Source: CAD feature listing. Evaluate the final solid. Frame: model axes, mm. A direction names the side the tool comes from. Round coordinates to 2 decimals unless told otherwise and drop trailing zeros. Write each loop counter-clockwise with the first axis right and the second up, starting at its lowest first coordinate (ties: lowest second). Pieces come first, ordered by that corner, then holes. Notation, with made-up numbers: (36.25, -16.5) - (78.25, -16.5) arc R21 ccw to (78.25, -3.5) - close; hole circle Ø7 at (17, -1). An arc over 180 degrees is marked (long way). Write item = value, one per line. Start each with the question number.
Solid Edge part; units mm, degrees
sketch "Sketch1" plane through (0, 0, 0) normal (0, 1, 0) x (-1, 0, 0)
  line L0 (-47.7348, -12.5) -> (4.2652, -12.5)
  line L1 (4.2652, -12.5) -> (4.2652, 12.5)
  line L2 (-47.7348, 12.5) -> (4.2652, 12.5)
  line L3 (-47.7348, 12.5) -> (-47.7348, -12.5)
  dimension "D1" = 4.2652
  dimension "D2" = 47.7348
extrude "Protrusion1" add sketch "Sketch1" along normal blind 202
sketch "Sketch2" plane through (0, 202, 0) normal (0, 1, 0) x (-1, 0, 0)
  line L0 (-37.7348, -12.5) -> (-5.7348, -12.5)
  arc A0 (-37.7348, -12.5) -> (-5.7348, -12.5) centre (-21.7348, -12.5) cw
  dimension "D1" = 37.7348
extrude "Cutout1" cut sketch "Sketch2" against normal up to next
hole "Hole_7" at (0.7348, 197, -12.5) direction (0, 0, 1) diameter 6.647 end up to next
hole "Hole1" at (42.7348, 197, -12.5) direction (0, 0, 1) diameter 6.647 end up to next
hole "Hole2" at (42.7348, 97, -12.5) direction (0, 0, 1) diameter 6.647 end up to next
hole "Hole3" at (0.7348, 97, -12.5) direction (0, 0, 1) diameter 6.647 end up to next
sketch "Sketch3" plane through (-4.2652, -75, 0) normal (-1, 0, 0) x (0, -1, 0)
  line L0 (-85, -12.5) -> (-117, -12.5)
  arc A0 (-117, -12.5) -> (-85, -12.5) centre (-101, -12.5) cw
  dimension "D1" = 85
extrude "Cutout2" cut sketch "Sketch3" against normal up to next
hole "Hole_11" at (0.7348, 47, -12.5) direction (0, 0, 1) diameter 6.647 end up to next
hole "Hole4" at (0.7348, 5, -12.5) direction (0, 0, 1) diameter 6.647 end up to next
hole "Hole_13" at (21.7348, 80, 12.5) direction (0, 0, -1) diameter 8.376 end up to next
hole "Hole5" at (21.7348, 175, 12.5) direction (0, 0, -1) diameter 8.376 end up to next
properties material "Stainless steel"
(1) Reachability of faces 1 (the cylindrical face through (0.88, 93.68, -0.18)), 2 (the cylindrical face through (5.664, 25.648, 3.496)) from +Z, -Z, +X, -X, +Y, -Y: full face, straight path, thin tool, end or side. Return the list, or none.
(2) Section D-D (y = 133.5). Return the cut outline in (x, z).
(3) Section B-B (z = -9.25). Count the separate pieces of the cut face and the enclosed holes in it, plus the area to 3 significant figures.
(4) Section A-A (y = 5). Return the cut outline in (x, z), plus the area to 3 significant figures.
(5) Section C-C (y = 97). Return the cut outline in (x, z).
(6) Ray query, L1, parallel to Y at x = 1, z = 9.5; L2, parallel to X at y = 80, z = 7; L3, parallel to X at y = 197, z = -4.75. Return the intervals inside material, ascending. Write a range as from..to.
(7) Contact query for flat-ended pins moving along their axis: P1, Ø1.5, axis at x = 26, y = 82, coming from the -Z side; P2, Ø2, axis at x = 33, y = 113, coming from the -Z side; P3, Ø10.5, axis at x = 0.73, y = 197, coming from the -Z side; P4, Ø11, axis at x = 21.73, y = 175, coming from the -Z side. Output: stop coordinate, or through.
(8) Pull-direction query (Y, two-part tool) for faces 3 (the flat face through (22, 202, 5)), 4 (the flat face through (22, 100, 12.5)), 5 (the cylindrical face through (40.713, 94.363, -0.175)); classes: +Y half, -Y half, draft (parallel to the pull), parting line (faces both ways), or undercut.
Solution:
q1.face_1 = +Z, -Z
q1.face_2 = -Z, -X
q2.outline = (-4.27, -12.5) - (5.73, -12.5) arc R16 cw to (37.73, -12.5) - (47.73, -12.5) - (47.73, 12.5) - (-4.27, 12.5) - close
q3.separate_pieces = 3
q3.enclosed_holes = 6
q3.area = 3,640 mm^2
q4.outline = (-4.27, -12.5) - (-2.59, -12.5) - (-2.59, 12.5) - (-4.27, 12.5) - close; (4.06, -12.5) - (5.73, -12.5) arc R16 cw to (37.73, -12.5) - (47.73, -12.5) - (47.73, 12.5) - (4.06, 12.5) - close
q4.area = 732 mm^2
q5.outline = (-4.27, -12.5) - (-2.59, -12.5) - (-2.59, 12.5) - (-4.27, 12.5) - close; (4.06, -12.5) - (5.73, -12.5) arc R16 cw to (37.73, -12.5) - (39.41, -12.5) - (39.41, 12.5) - (4.06, 12.5) - close; (46.06, -12.5) - (47.73, -12.5) - (47.73, 12.5) - (46.06, 12.5) - close
q6.L1 = 0..1.69, 8.31..43.69, 50.31..93.69, 100.31..193.69, 200.31..202
q6.L2 = -4.27..17.55, 25.92..47.73
q6.L3 = -4.27..-2.59, 4.06..7.74, 35.73..39.41, 46.06..47.73
q7.P1 = 2.69
q7.P2 = -2.23
q7.P3 = -12.5
q7.P4 = 2.52
q8.face_3 = +Y half
q8.face_4 = draft
q8.face_5 = undercut
